Build history of the part. All positions in model axes, mm. Give positions to 0.01 mm unless a question says otherwise; leave off trailing zeros. Order: outer loops, then holes, each group sorted by start corner. A loop starts at its lowest first (then second) coordinate and runs counter-clockwise, first axis right, second up. Notation, with made-up numbers: (6, 31) - (56, 31) arc R25 cw to (56, 52) - close; hole circle Ø3 at (38, -11). An arc over 180 degrees is marked (long way). Use a Markdown table: item, result. Add a question column.
(1) Wall check: line 1 (Z direction, x = 128.5, y = 3.65); line 2 (X direction, y = 2.65, z = -127). Give the ranges that are in metal, low to high.
(2) Flat gauge pins, fed straight in: pin 1 (1 mm diameter, centred on y = 1.5, z = -64.5, fed in from +X); pin 2 (1.8 mm diameter, centred on y = 2.5, z = -4.5, fed in from +X); pin 3 (1.5 mm diameter, centred on x = 112.5, z = -165.5, fed in from -Y); pin 4 (3 mm diameter, centred on x = 93, y = 2.5, fed in from +Z). Where does each tip first touch, or does it go through?
(3) Slice it at B-B (z = -141). Write the cut outline in (x, y).
(4) Slice it at A-A (x = 132). Write the cut outline in (y, z), then the cut area to 3 significant figures.
from build123d import *

# Parameters (mm, degrees)
SKETCH1_W           = 150
SKETCH1_H           = 200
BOSS_EXTRUDE1_DEPTH = 6
SKETCH2_W           = 25
SKETCH2_H           = 6
SKETCH2_W_2         = 6
SKETCH2_H_2         = 40
CUT_EXTRUDE1_DEPTH  = 6


with BuildPart() as part:
    # Sketch1 → Boss-Extrude1 (new body)
    with BuildSketch(Plane(origin=(0, 0, 0), x_dir=(1, 0, 0), z_dir=(0, 1, 0))):
        with Locations((75, 100)):
            Rectangle(SKETCH1_W, SKETCH1_H)
    extrude(amount=BOSS_EXTRUDE1_DEPTH)

    # Sketch2 → Cut-Extrude1 (cut)
    with BuildSketch(Plane(origin=(0, 6, 0), x_dir=(1, 0, 0), z_dir=(0, 1, 0))):
        with Locations((37.5, 3)):
            Rectangle(SKETCH2_W, SKETCH2_H)
        with Locations((87.5, 3)):
            Rectangle(SKETCH2_W, SKETCH2_H)
        with Locations((137.5, 3)):
            Rectangle(SKETCH2_W, SKETCH2_H)
        with Locations((37.5, 197)):
            Rectangle(SKETCH2_W, SKETCH2_H)
        with Locations((87.5, 197)):
            Rectangle(SKETCH2_W, SKETCH2_H)
        with Locations((137.5, 197)):
            Rectangle(SKETCH2_W, SKETCH2_H)
        with Locations((3, 140)):
            Rectangle(SKETCH2_W_2, SKETCH2_H_2)
        with Locations((147, 140)):
            Rectangle(SKETCH2_W_2, SKETCH2_H_2)
        with Locations((147, 60)):
            Rectangle(SKETCH2_W_2, SKETCH2_H_2)
        with Locations((3, 60)):
            Rectangle(SKETCH2_W_2, SKETCH2_H_2)
    extrude(amount=-CUT_EXTRUDE1_DEPTH, mode=Mode.SUBTRACT)


solid = part.part
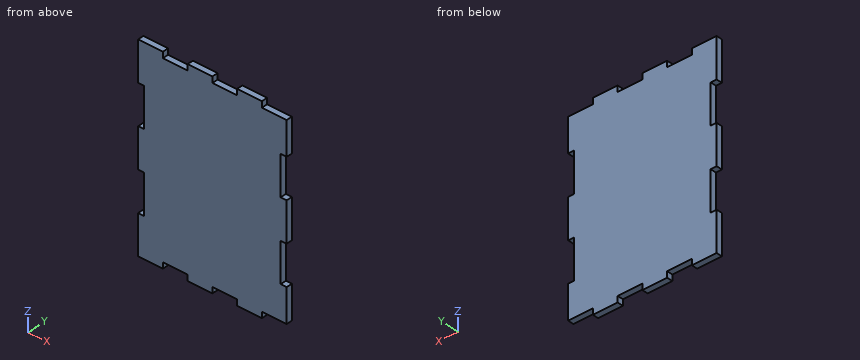
Solution:
| question | item | result |
|---|---|---|
| 1 | line 1 | -194 to -6 |
| 1 | line 2 | 6 to 144 |
| 2 | pin 1 | x = 144 |
| 2 | pin 2 | x = 125 |
| 2 | pin 3 | y = 0 |
| 2 | pin 4 | z = -6 |
| 3 | outline | (6, 0) - (144, 0) - (144, 6) - (6, 6) - close |
| 4 | outline | (0, -194) - (6, -194) - (6, -6) - (0, -6) - close |
| 4 | area | 1,130 mm2 |
